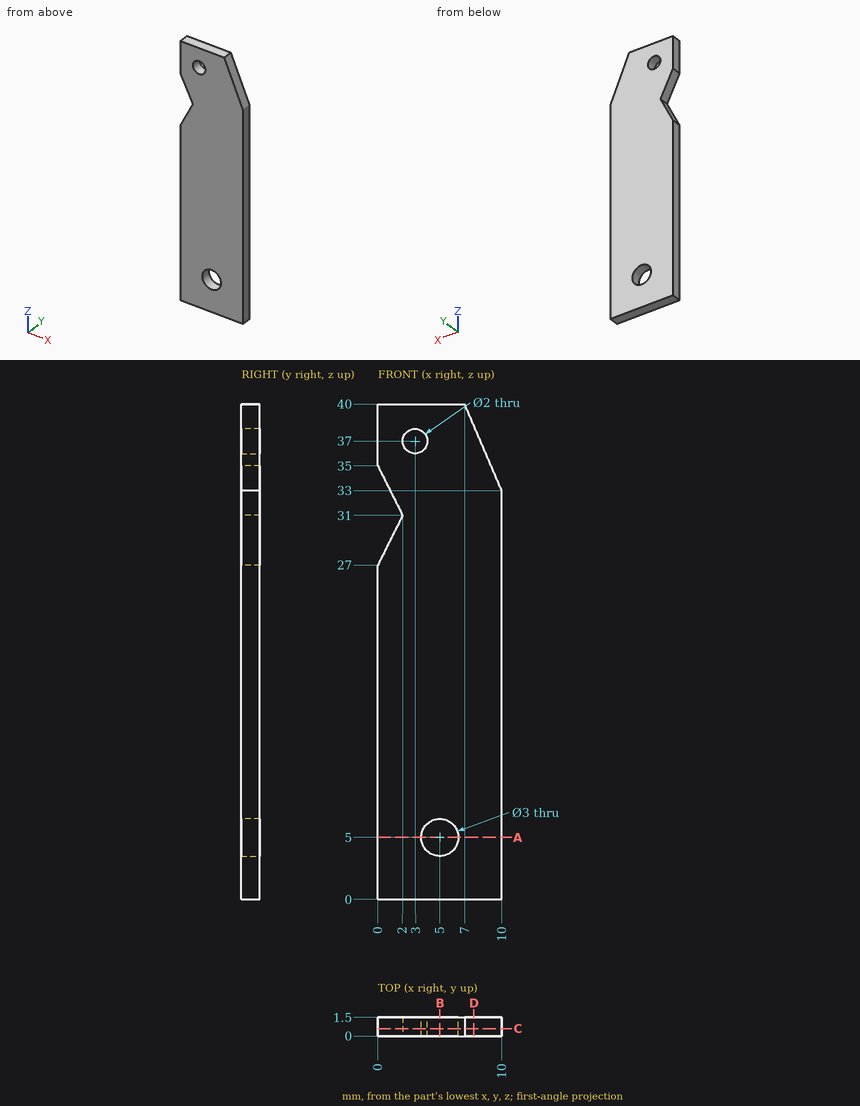
Geometry check sheet. Reference: drawing and pictorial views, mm from the part's lowest x, y, z. Give positions to 0.01 mm unless a question says otherwise; leave off trailing zeros. Write each loop counter-clockwise with the first axis right and the second up, starting at its lowest first coordinate (ties: lowest second). Pieces come first, ordered by that corner, then holes. Notation, with made-up numbers: (82.5, -2) -> (107.5, -2) arc R17 ccw to (107.5, 5) -> close; hole circle Ø3 at (-39, 12.5). An arc over 180 degrees is marked (long way). One line per question, with ' | ' between items.
Item 1: Scan lines: line 1 along X through (y, z) = (0.55, 5); line 2 along X through (y, z) = (0.3, 37); line 3 along Z through (x, y) = (6.25, 1). Record each from-to range of solid material in increasing order.
Determined:
line 1: 0 to 3.5, 6.5 to 10 | line 2: 0 to 2, 4 to 8.29 | line 3: 0 to 4.17, 5.83 to 40
Item 2: Sectioned sample at A-A, the plane z = 5. Record the boundary of the cut face in (x, y).
Determined:
outline: (0, 0) -> (3.5, 0) -> (3.5, 1.5) -> (0, 1.5) -> close; (6.5, 0) -> (10, 0) -> (10, 1.5) -> (6.5, 1.5) -> close
Item 3: Sectioned sample at C-C, the plane y = 0.6. Record the boundary of the cut face in (x, z).
Determined:
outline: (0, 0) -> (10, 0) -> (10, 33) -> (7, 40) -> (0, 40) -> (0, 35) -> (2, 31) -> (0, 27) -> close; hole circle Ø2 at (3, 37); hole circle Ø3 at (5, 5)
Item 4: Sectioned sample at D-D, the plane x = 7.75. Record the boundary of the cut face in (y, z), plus the area to 3 significant figures.
Determined:
outline: (0, 0) -> (1.5, 0) -> (1.5, 38.25) -> (0, 38.25) -> close | area: 57.4 mm^2
Item 5: Sectioned sample at B-B, the plane x = 5. Record the boundary of the cut face in (y, z).
Determined:
outline: (0, 0) -> (1.5, 0) -> (1.5, 3.5) -> (0, 3.5) -> close; (0, 6.5) -> (1.5, 6.5) -> (1.5, 40) -> (0, 40) -> close
